Job drawing, mm, ordinate dimensions from the low corner. One solid piece. Round coordinates to 2 decimals unless told otherwise and drop trailing zeros. Order: outer loops, then holes, each group sorted by start corner. A loop starts at its lowest first (then second) coordinate and runs counter-clockwise, first axis right, second up. Notation, with made-up numbers: (67.25, 85.25) -> (100.25, 85.25) arc R12 cw to (100.25, 102.25) -> close; hole circle Ø7 at (22.25, 20). An arc over 180 degrees is marked (long way). Return JSON: item names as keys, results as strings. Group by question number.
Q1. Probe line 1 along X through (y, z) = (27.5, 1.3); line 2 along X through (y, z) = (37.5, 0.3); line 3 along Y through (x, z) = (70, 1.1). List the from-to ranges inside material, lowest first.
Q2. Cut at C-C (x = 30). Write the cut outline in (y, z).
Q3. Mould opens along Z. For the marked faces 1 and 2 say: +Z half, -Z half, draft (parallel to the pull), parting line (faces both ways), or undercut.
Q4. Cut at D-D (y = 58). Write the cut outline in (x, z), then the cut area to 3 significant figures.
Q5. Cut at A-A (x = 50). Write the cut outline in (y, z).
Q6. Cut at B-B (z = 0.95). Write the cut outline in (x, y).
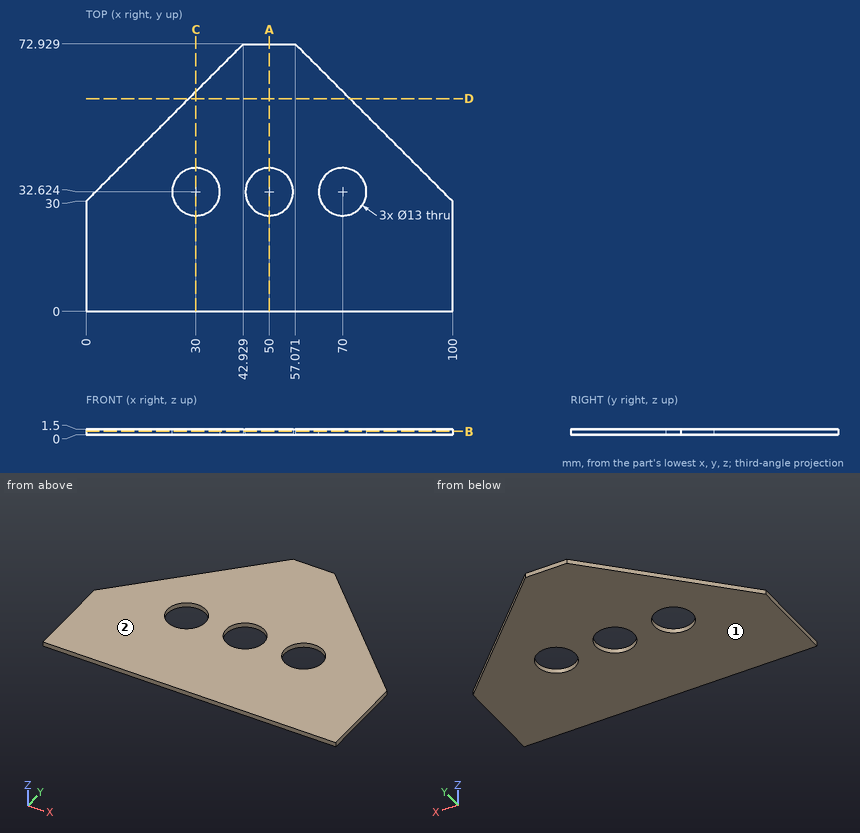
Solution:
{
 "1": {"line 1": "x = 0 to 26, 34 to 46, 54 to 66, 74 to 100", "line 2": "x = 7.5 to 25.7, 34.3 to 45.7, 54.3 to 65.7, 74.3 to 92.5", "line 3": "y = 0 to 26.12, 39.12 to 60"},
 "2": {"outline": "(0, 0) -> (26.12, 0) -> (26.12, 1.5) -> (0, 1.5) -> close; (39.12, 0) -> (60, 0) -> (60, 1.5) -> (39.12, 1.5) -> close"},
 "3": {"face 1": "-Z half", "face 2": "+Z half"},
 "4": {"outline": "(28, 0) -> (72, 0) -> (72, 1.5) -> (28, 1.5) -> close", "area": "66.0 mm²"},
 "5": {"outline": "(0, 0) -> (26.12, 0) -> (26.12, 1.5) -> (0, 1.5) -> close; (39.12, 0) -> (72.93, 0) -> (72.93, 1.5) -> (39.12, 1.5) -> close"},
 "6": {"outline": "(0, 0) -> (100, 0) -> (100, 30) -> (57.07, 72.93) -> (42.93, 72.93) -> (0, 30) -> close; hole circle Ø13 at (30, 32.62); hole circle Ø13 at (50, 32.62); hole circle Ø13 at (70, 32.62)"}
}
